Autodesk Inventor part; units mm, degrees
ref_plane "YZ Plane" through (0, 0, 0) normal (1, 0, 0) x (0, 1, 0)
ref_plane "XZ Plane" through (0, 0, 0) normal (0, 1, 0) x (-1, 0, 0)
ref_plane "XY Plane" through (0, 0, 0) normal (0, 0, 1) x (1, 0, 0)
sketch "Sketch1" plane through (0, 0, 0) normal (0, 0, 1) x (1, 0, 0)
  line L0 (-40.3774, 59.0566) -> (39.6226, 59.0566)
  line L1 (39.6226, 59.0566) -> (39.6226, 159.0566)
  line L2 (39.6226, 159.0566) -> (-40.3774, 159.0566)
  line L3 (-40.3774, 159.0566) -> (-40.3774, 59.0566)
  point P0 (0, 0)
  dimension "d0" = 80
  dimension "d1" = 100
extrude "Extrusion1" add sketch "Sketch1" along normal blind 1800
sketch "Sketch2" plane through (39.6226, 59.0566, 0) normal (1, 0, 0) x (0, 0, -1)
  line L0 (403.6788, -347.1669) -> (-104.7907, 650.76)
  line L1 (-104.7907, 650.76) -> (-128.8479, 638.5023)
  line L2 (379.6216, -359.4246) -> (-128.8479, 638.5023)
  line L3 (403.6788, -347.1669) -> (379.6216, -359.4246)
  line L4 (0, 0) -> (-1800, 0)
  line L5 (0, 0) -> (-117.0664, 229.7556)
  line L6 (-112.2326, 0) -> (-212.1687, 196.1355)
  line L7 (0, 0) -> (-112.2326, 0)
  line L8 (0, 0) -> (0, 100)
  line L9 (0, 100) -> (-1800, 100)
  line L10 (-163.1852, 100) -> (-50.9526, 100)
  point P0 (0, -59.0566)
  dimension "d4" = 100
extrude "Extrusion2" cut sketch "Sketch2" against normal blind 25 contours L4 L6 L9 L5
sketch "Sketch3" plane through (39.6226, 59.0566, 0) normal (1, 0, 0) x (0, 0, -1)
  line L0 (-50.9526, 100) -> (0, 0)
  line L1 (0, 0) -> (0, 100)
  line L2 (0, 100) -> (-50.9526, 100)
  point P0 (0, -59.0566)
sketch "Sketch4" plane through (39.6226, 59.0566, 0) normal (1, 0, 0) x (0, 0, -1)
  point P0 (0, -59.0566)
extrude "Extrusion3" cut sketch "Sketch3" against normal blind 100
sketch "Sketch5" plane through (-40.3774, 59.0566, 1800) normal (-1, 0, 0) x (0, 0, 1)
  line L0 (-1687.7674, 0) -> (-1636.8148, 100)
  line L1 (-1749.0474, 100) -> (-1800, 0)
  line L2 (-1800, 0) -> (0, 0)
  line L3 (0, 100) -> (0, 0)
  line L4 (-1749.0474, 100) -> (0, 100)
  point P0 (-1800, -59.0566)
  point P1 (-1687.7674, 0)
extrude "Extrusion4" cut sketch "Sketch5" against normal blind 25 contours L2 L1 L4 L0
properties part number "poutre100x80" material "Wood (Birch)"
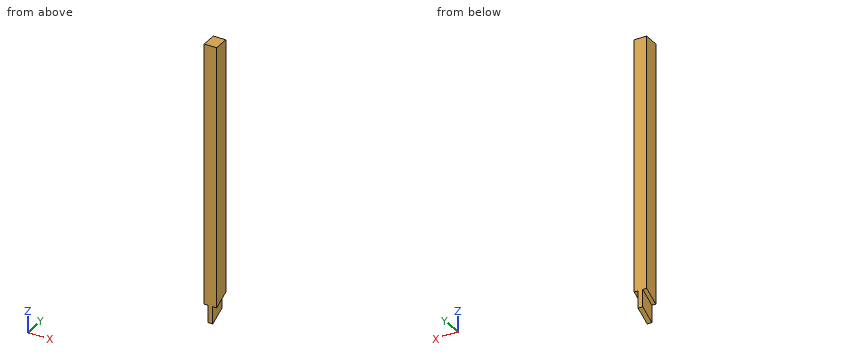
Work out the finished part from the listing and answer in its coordinate system (mm). Coordinates: 2 decimals unless noted, no trailing zeros. Order: outer loops, then holes, each group sorted by start corner. A loop starts at its lowest first (then second) coordinate and runs counter-clockwise, first axis right, second up. Notation, with made-up numbers: (0.25, 83) - (18.25, 83) arc R14 cw to (18.25, 94) - close; hole circle Ø4 at (2.25, 29.5). An arc over 180 degrees is marked (long way). Answer as a JSON object with one key per item and string values.
1. Consider line 1 (Z direction, x = 35, y = 151.5); line 2 (Z direction, x = -36.5, y = 140). Determine where each line is inside the solid, lowest interval first.
Output values:
{"line 1": "z = 159.33 to 1800", "line 2": "z = 153.48 to 1800"}
2. This flat-tipped pin is pushed along its axis until it touches: P1, Ø8, axis at x = -12, y = 124, coming from the -Z side. Where does it stop, or does it pass through?
Output values:
{"P1": "stops at z = 31.05"}
3. Find section A-A on y = 133.5. Determine the outline of the cut face in (x, z), plus the area to 3 significant figures.
Output values:
{"outline": "(-40.38, 150.16) - (-15.38, 150.16) - (-15.38, 37.93) - (14.62, 37.93) - (14.62, 150.16) - (39.62, 150.16) - (39.62, 1800) - (-40.38, 1800) - close", "area": "135,000 mm²"}
